from build123d import *

# Parameters (mm, degrees)
SKETCH1_R            = 3.25
SKETCH1_R_2          = 2.25
SKETCH1_R_3          = 25
SKETCH1_W            = 18
SKETCH1_H            = 25.4
BOSS_EXTRUDE1_DEPTH  = 15
SKETCH2_W            = 7.5
SKETCH2_H            = 12
BLOWER_OPENING_DEPTH = 20


with BuildPart() as part:
    # Sketch1 → Boss-Extrude1 (new body)
    # profile 1 of 11: a face of its own
    with BuildSketch(Plane(origin=(0, 0, 0), x_dir=(1, 0, 0), z_dir=(0, 1, 0))):
        with Locations((-20.1, 20.1)):
            Circle(SKETCH1_R)
        with Locations(Location((-20.1, 20.1, 0), (0, 0, 270))):
            Circle(SKETCH1_R_2, mode=Mode.SUBTRACT)
    # profile 2 of 11: a face of its own
    with BuildSketch(Plane(origin=(0, 0, 0), x_dir=(1, 0, 0), z_dir=(0, 1, 0))):
        with BuildLine():
            ThreePointArc((-20.435592731, 15.839398654), (-20.146067758, 15.214298861), (-20.329518762, 14.550280647))
            ThreePointArc((-20.329518762, 14.550280647), (-17.67766953, 17.67766953), (-14.550280647, 20.329518762))
            ThreePointArc((-14.550280647, 20.329518762), (-15.214298861, 20.146067758), (-15.839398654, 20.435592731))
            Line((-15.839398654, 20.435592731), (-17.801902961, 22.398097039))
            ThreePointArc((-17.801902961, 22.398097039), (-17.097391519, 21.343721155), (-16.85, 20.1))
            ThreePointArc((-16.85, 20.1), (-18.856278845, 17.097391519), (-22.398097039, 17.801902961))
            Line((-22.398097039, 17.801902961), (-20.435592731, 15.839398654))
        make_face()
    # profile 3 of 11: a face of its own
    with BuildSketch(Plane(origin=(0, 0, 0), x_dir=(1, 0, 0), z_dir=(0, 1, 0))):
        with BuildLine():
            ThreePointArc((20.329518762, -14.550280647), (17.67766953, -17.67766953), (14.550280647, -20.329518762))
            ThreePointArc((14.550280647, -20.329518762), (15.214298861, -20.146067758), (15.839398654, -20.435592731))
            Line((15.839398654, -20.435592731), (17.801902961, -22.398097039))
            ThreePointArc((17.801902961, -22.398097039), (17.801902961, -17.801902961), (22.398097039, -17.801902961))
            Line((22.398097039, -17.801902961), (20.435592731, -15.839398654))
            ThreePointArc((20.435592731, -15.839398654), (20.146067758, -15.214298861), (20.329518762, -14.550280647))
        make_face()
    # profile 4 of 11: a face of its own
    with BuildSketch(Plane(origin=(0, 0, 0), x_dir=(1, 0, 0), z_dir=(0, 1, 0))):
        with Locations((20.1, -20.1)):
            Circle(SKETCH1_R)
        with Locations(Location((20.1, -20.1, 0), (0, 0, 270))):
            Circle(SKETCH1_R_2, mode=Mode.SUBTRACT)
    # profile 5 of 11: a face of its own
    with BuildSketch(Plane(origin=(0, 0, 0), x_dir=(1, 0, 0), z_dir=(0, 1, 0))):
        with BuildLine():
            ThreePointArc((-20.329518762, 14.550280647), (-23.980330253, 7.067089993), (-24.971183392, -1.2))
            Line((-24.971183392, -1.2), (-9.7, -1.2))
            Line((-9.7, -1.2), (-9.7, -23.041484327))
            ThreePointArc((-9.7, -23.041484327), (2.778487879, -24.845120348), (14.550280647, -20.329518762))
            ThreePointArc((14.550280647, -20.329518762), (17.67766953, -17.67766953), (20.329518762, -14.550280647))
            ThreePointArc((20.329518762, -14.550280647), (23.803759882, -7.640747049), (25, 0))
            ThreePointArc((25, 0), (11.428975978, 22.234624082), (-14.550280647, 20.329518762))
            ThreePointArc((-14.550280647, 20.329518762), (-17.67766953, 17.67766953), (-20.329518762, 14.550280647))
        make_face()
    # profile 6 of 11: a face of its own
    with BuildSketch(Plane(origin=(0, 0, 0), x_dir=(1, 0, 0), z_dir=(0, 1, 0))):
        with BuildLine():
            Line((-9.7, -1.2), (-24.971183392, -1.2))
            ThreePointArc((-24.971183392, -1.2), (-20.488663911, -14.325315045), (-9.7, -23.041484327))
            Line((-9.7, -23.041484327), (-9.7, -1.2))
        make_face()
    # profile 7 of 11: a face of its own
    with BuildSketch(Plane(origin=(0, 0, 0), x_dir=(1, 0, 0), z_dir=(0, 1, 0))):
        with BuildLine():
            ThreePointArc((-20.329518762, 14.550280647), (-23.980330253, 7.067089993), (-24.971183392, -1.2))
            Line((-24.971183392, -1.2), (-9.7, -1.2))
            Line((-9.7, -1.2), (-9.7, -23.041484327))
            ThreePointArc((-9.7, -23.041484327), (2.778487879, -24.845120348), (14.550280647, -20.329518762))
            ThreePointArc((14.550280647, -20.329518762), (17.67766953, -17.67766953), (20.329518762, -14.550280647))
            ThreePointArc((20.329518762, -14.550280647), (23.803759882, -7.640747049), (25, 0))
            ThreePointArc((25, 0), (11.428975978, 22.234624082), (-14.550280647, 20.329518762))
            ThreePointArc((-14.550280647, 20.329518762), (-17.67766953, 17.67766953), (-20.329518762, 14.550280647))
        make_face()
    # profile 8 of 11: a face of its own
    with BuildSketch(Plane(origin=(0, 0, 0), x_dir=(1, 0, 0), z_dir=(0, 1, 0))):
        with BuildLine():
            Line((-9.7, -1.2), (-24.971183392, -1.2))
            ThreePointArc((-24.971183392, -1.2), (-20.488663911, -14.325315045), (-9.7, -23.041484327))
            Line((-9.7, -23.041484327), (-9.7, -1.2))
        make_face()
    # profile 9 of 11: a face of its own
    with BuildSketch(Plane(origin=(0, 0, 0), x_dir=(1, 0, 0), z_dir=(0, 1, 0))):
        Circle(SKETCH1_R_3)
    # profile 10 of 11: a face of its own
    with BuildSketch(Plane(origin=(0, 0, 0), x_dir=(1, 0, 0), z_dir=(0, 1, 0))):
        with Locations((-18.7, -13.9)):
            Rectangle(SKETCH1_W, SKETCH1_H)
    # profile 11 of 11: a face of its own
    with BuildSketch(Plane(origin=(0, 0, 0), x_dir=(1, 0, 0), z_dir=(0, 1, 0))):
        with BuildLine():
            ThreePointArc((-20.329518762, 14.550280647), (-24.739386117, 7.014235726), (-27.7, -1.2))
            Line((-27.7, -1.2), (-24.971183392, -1.2))
            ThreePointArc((-24.971183392, -1.2), (-23.980330253, 7.067089993), (-20.329518762, 14.550280647))
        make_face()
    extrude(amount=BOSS_EXTRUDE1_DEPTH)

    # Sketch2 → blower opening (cut)
    with BuildSketch(Plane.XY.offset(26.6)):
        with Locations((-22.45, 7.5)):
            Rectangle(SKETCH2_W, SKETCH2_H)
        with Locations((-14.95, 7.5)):
            Rectangle(SKETCH2_W, SKETCH2_H)
    extrude(amount=-BLOWER_OPENING_DEPTH, mode=Mode.SUBTRACT)


solid = part.part
CAD build for the part. Positions are in the model's coordinates, mm. A direction names the side the tool comes from. Round coordinates to 2 decimals unless told otherwise and drop trailing zeros. Order: outer loops, then holes, each group sorted by start corner. A loop starts at its lowest first (then second) coordinate and runs counter-clockwise, first axis right, second up. Notation, with made-up numbers: (36, 15) -> (56, 15) arc R20 cw to (56, 41) -> close; hole circle Ø7 at (52.5, 74). An arc over 180 degrees is marked (long way). Write item = value, one per line. Start each with the question number.
(1) Pin check, flat tips, straight feed: P1, Ø1.5, axis at x = -17, y = 7.5, coming from the -Z side; P2, Ø4, axis at y = 3.5, z = -19.5, coming from the +X side; P3, Ø1, axis at y = 12.5, z = -12.5, coming from the +X side. Stop position of each tip, or through.
(2) Cut at C-C, the plane z = -11.5. List the corners of the cut face in (x, y).
(3) Which spindle directions (+Z, -Z, +X, -X, +Y, -Y) get a long thin tool onto all of the face, cutting with end or side? Do faces 4 (the cylindrical face through (-24.7, 7.4, -7.1)), 5 (the cylindrical face through (-22.347, 7.395, -22.448)), 6 (the flat face through (-19, 8, 6.6)), 7 (the flat face through (-9.7, 7, 25)), 8 (the flat face through (21.431, 7.395, 16.834)). Say none if no direction does.
(4) Cut at A-A, the plane y = 8. List the corners of the cut face in (x, z), then the cut area to 3 significant figures.
(5) Cut at B-B, the plane x = 9.5. List the corners of the cut face in (y, z).
(6) Probe line 1 (X direction, y = 3.5, z = 20.1); line 2 (X direction, y = 4.5, z = -20); line 3 (X direction, y = 9.25, z = -20.1). List the from-to ranges inside material, lowest first. Write a range as [from, to].
(7) Pull direction Y, two halves, no side cores. Call faces 1 (the flat face through (-19, 1.5, 17)), 2 (the flat face through (-21.431, 7.395, -16.834)), 3 (the flat face through (-2, 0, 0)): released by +Y, released by -Y, zero draft, split by the parting line, or undercut.
Model answer:
q1.P1 = -22.35
q1.P2 = 17.85
q1.P3 = 21.93
q2.outline = (-22.34, 0) -> (22.2, 0) -> (22.2, 15) -> (-22.34, 15) -> close
q3.face_4 = -X, +Y, -Y
q3.face_5 = +Y, -Y
q3.face_6 = +Z
q3.face_7 = +Z, +Y, -Y
q3.face_8 = +X, +Y, -Y
q4.outline = (-27.7, 1.2) arc R47.65 ccw to (-20.33, -14.55) arc R1 cw to (-20.44, -15.84) -> (-22.4, -17.8) arc R3.25 ccw to (-17.8, -22.4) -> (-15.84, -20.44) arc R1 cw to (-14.55, -20.33) arc R25 ccw to (20.33, 14.55) arc R1 cw to (20.44, 15.84) -> (22.4, 17.8) arc R3.25 ccw to (17.8, 22.4) -> (15.84, 20.44) arc R1 cw to (14.55, 20.33) arc R25 ccw to (-9.7, 23.04) -> (-9.7, 26.6) -> (-11.2, 26.6) -> (-11.2, 6.6) -> (-26.2, 6.6) -> (-26.2, 26.6) -> (-27.7, 26.6) -> close; hole circle Ø4.5 at (-20.1, -20.1); hole circle Ø4.5 at (20.1, 20.1)
q4.area = 1,950 mm2
q5.outline = (0, -23.12) -> (15, -23.12) -> (15, 23.12) -> (0, 23.12) -> close
q6.line_1 = [-27.7, -26.2], [-11.2, 17.85], [22.35, 23.35]
q6.line_2 = [-23.35, -22.35], [-17.85, 15]
q6.line_3 = [-23.35, -22.35], [-17.85, 14.87]
q7.face_1 = undercut
q7.face_2 = zero draft
q7.face_3 = released by -Y
